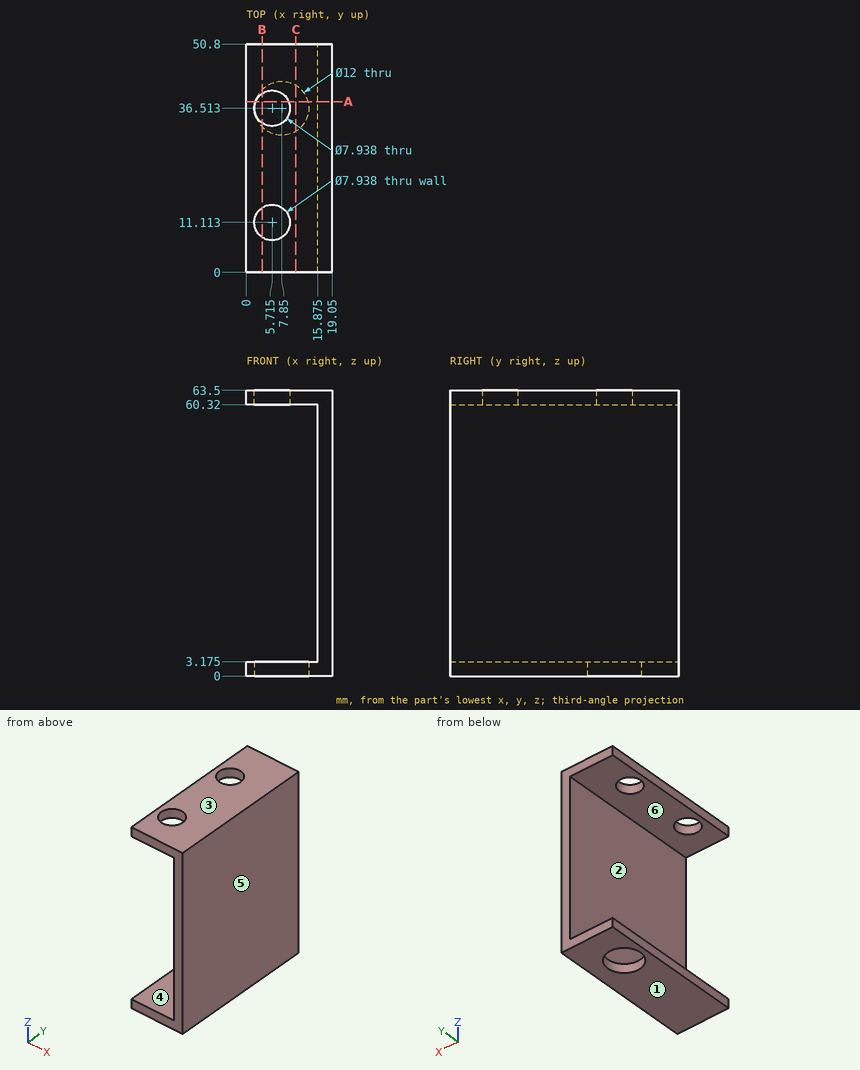
Geometry check sheet. Reference: drawing and pictorial views, mm from the part's lowest x, y, z. A direction names the side the tool comes from. Round coordinates to 2 decimals unless told otherwise and drop trailing zeros. Loops run counter-clockwise (first coordinate to the right, second up) from the corner with the lowest first, then second, coordinate; pieces in that order, holes last. Notation, with made-up numbers: (64, 0.25) - (114, 0.25) arc R19 ccw to (114, 17.25) - close; hole circle Ø8 at (32.25, 86). An arc over 180 degrees is marked (long way). Write item = value, one per line. Start each with the question number.
Q1. Release check for a two-part mould opening along Z. For the marked faces 1, 2, 3 and 4 record: pulls with the +Z half, pulls with the -Z half, needs draft (parallel to the pull), parting line crosses it, or undercut.
Q2. Thickness scan on L1, parallel to Z at x = 8.75, y = 3 (1 decimal); L2, parallel to Y at x = 7.85, z = 0.7; L3, parallel to Z at x = 8, y = 32.5. Record the ranges inside material, lowest first.
Q3. Section check A-A (y = 38). Count the separate pieces of the cut face and the enclosed holes in it, plus the area to 3 significant figures.
Q4. Depth check by flat-ended pin: P1, Ø1.5, axis at x = 14.5, z = 43.5, coming from the +Y side; P2, Ø6, axis at y = 8, z = 7, coming from the -X side (1 decimal); P3, Ø1, axis at x = 3, y = 34, coming from the -Z side. Enter the tip coordinate at first touch or a pass-through.
Q5. Section check C-C (x = 11). Record the boundary of the cut face in (y, z) (1 decimal).
Q6. Section check B-B (x = 3.5). Record the boundary of the cut face in (y, z) (1 decimal).
Q7. Access from +Z, -Z, +X, -X, +Y, -Y to the whole of each face (thin tool, end or side, straight path). Record for the marked faces 5 and 6.
Derived:
q1.face_1 = pulls with the -Z half
q1.face_2 = undercut
q1.face_3 = pulls with the +Z half
q1.face_4 = undercut
q2.L1 = 0 to 3.2, 60.3 to 63.5
q2.L2 = 0 to 30.51, 42.51 to 50.8
q2.L3 = 60.32 to 63.5
q3.separate_pieces = 3
q3.enclosed_holes = 0
q3.area = 242 mm^2
q4.P1 = through
q4.P2 = 15.9
q4.P3 = 60.32
q5.outline = (0, 0) - (31.4, 0) - (31.4, 3.2) - (0, 3.2) - close; (0, 60.3) - (50.8, 60.3) - (50.8, 63.5) - (0, 63.5) - close; (41.6, 0) - (50.8, 0) - (50.8, 3.2) - (41.6, 3.2) - close
q6.outline = (0, 0) - (32.4, 0) - (32.4, 3.2) - (0, 3.2) - close; (0, 60.3) - (7.8, 60.3) - (7.8, 63.5) - (0, 63.5) - close; (14.4, 60.3) - (33.2, 60.3) - (33.2, 63.5) - (14.4, 63.5) - close; (39.8, 60.3) - (50.8, 60.3) - (50.8, 63.5) - (39.8, 63.5) - close; (40.6, 0) - (50.8, 0) - (50.8, 3.2) - (40.6, 3.2) - close
q7.face_5 = +Z, -Z, +X, +Y, -Y
q7.face_6 = -X, +Y, -Y
